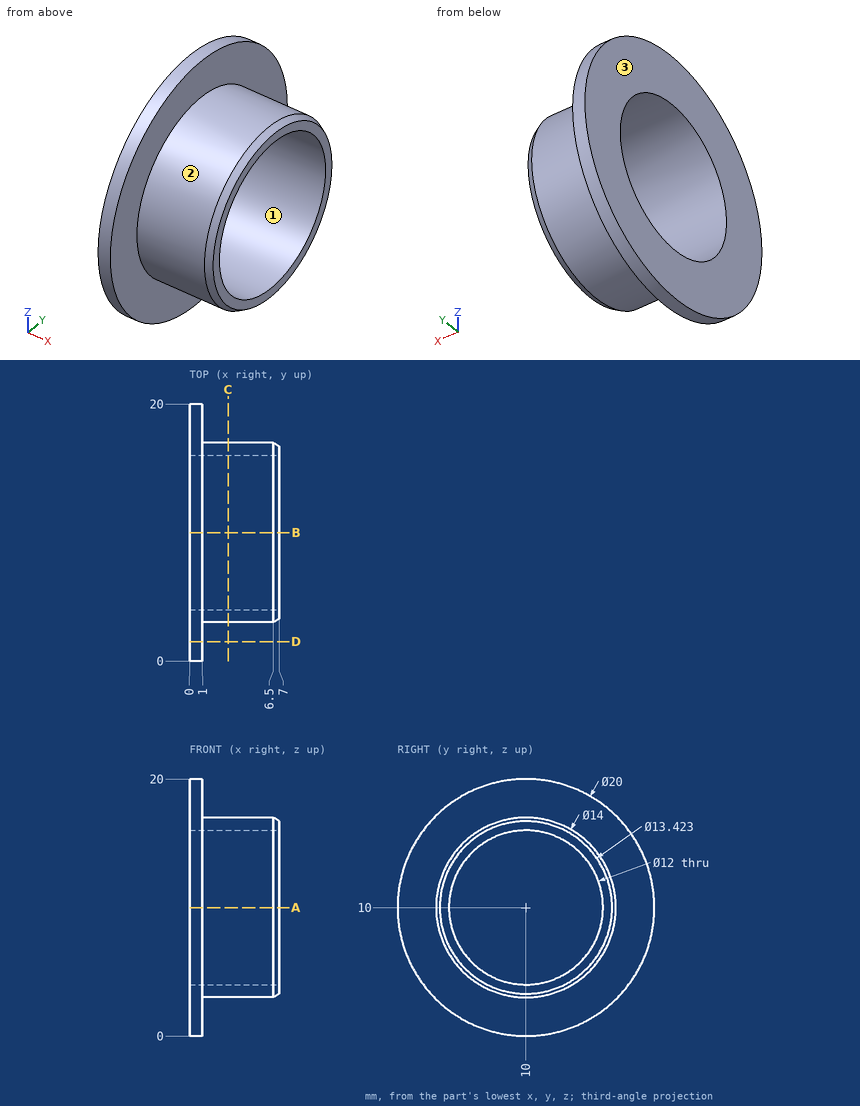
Check sheet for the drawn part. Datum: minimum x, y, z corner. Units: mm. Round coordinates to 2 decimals unless told otherwise and drop trailing zeros. Loops run counter-clockwise (first coordinate to the right, second up) from the corner with the lowest first, then second, coordinate; pieces in that order, holes last. Notation, with made-up numbers: (53, 52.5) - (85, 52.5) arc R22 cw to (85, 89.5) - close; hole circle Ø7 at (-9, -32). An arc over 180 degrees is marked (long way). Write each question's results on one line, items separated by ' | '. Start each with the question number.
Q1. Gauge pin test, flat ends, axial feed: P1, Ø1.5, axis at x = 3.5, z = 7.5, coming from the -Y side; P2, Ø11, axis at y = 10, z = 10, coming from the +X side; P3, Ø2, axis at x = 4.5, z = 5, coming from the +Y side (1 decimal); P4, Ø1.5, axis at x = 1, z = 8, coming from the -Y side. Record the tip position at first contact, or that the pin passes through.
Q2. Cross-section at C-C on x = 3. Enter the section's corners in (y, z).
Q3. Cross-section at D-D on y = 1.5. Enter the section's corners in (x, z).
Q4. Thickness scan on line 1 (Z direction, x = 3, y = 10); line 2 (X direction, y = 18.75, z = 5.25); line 3 (Y direction, x = 0.5, z = 18). Record the ranges inside material, lowest first. Write a range as [from, to].
Q5. Release check for a two-part mould opening along Y. For the marked faces 1, 2 and 3 record: +Y half, -Y half, draft (parallel to the pull), parting line (faces both ways), or undercut.
Q6. Cross-section at A-A on z = 10. Enter the section's corners in (x, y).
Answers below:
1) P1: stops at y = 3.22 | P2: passes through | P3: stops at y = 15.7 | P4: stops at y = 0.08
2) outline: circle Ø14 at (10, 10); hole circle Ø12 at (10, 10)
3) outline: (0, 4.73) - (1, 4.73) - (1, 15.27) - (0, 15.27) - close
4) line 1: z = [3, 4], [16, 17] | line 2: x = [0, 1] | line 3: y = [4, 16]
5) face 1: undercut | face 2: parting line | face 3: draft
6) outline: (0, 0) - (1, 0) - (1, 3) - (6.5, 3) - (7, 3.29) - (7, 4) - (0, 4) - close; (0, 16) - (7, 16) - (7, 16.71) - (6.5, 17) - (1, 17) - (1, 20) - (0, 20) - close
